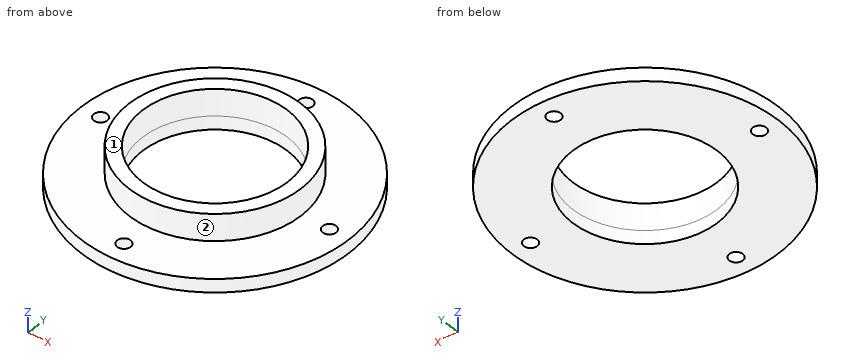
Autodesk Inventor part; units mm, degrees
ref_plane "YZ Plane" through (0, 0, 0) normal (1, 0, 0) x (0, 1, 0)
ref_plane "XZ Plane" through (0, 0, 0) normal (0, 1, 0) x (-1, 0, 0)
ref_plane "XY Plane" through (0, 0, 0) normal (0, 0, 1) x (1, 0, 0)
sketch "Boceto1" plane through (0, 0, 0) normal (0, 0, 1) x (1, 0, 0)
  circle A0 centre (0, 0) radius 16.26
  circle A1 centre (0, 0) radius 19.26
  dimension "d0" = 32.52
  dimension "d1" = 3
extrude "Extrusión1" add sketch "Boceto1" along normal blind 6
sketch "Boceto2" plane through (0, 0, 0) normal (0, 0, -1) x (-1, 0, 0)
  circle A0 centre (0, 0) radius 30
  circle A1 centre (0, 0) radius 16.26
  dimension "d4" = 60
extrude "Extrusión2" add sketch "Boceto2" along normal blind 3
sketch "Boceto3" plane through (0, 0, 0) normal (0, 0, 1) x (1, 0, 0)
  circle A0 centre (0, 0) radius 30
  circle A1 centre (0, 25.5) radius 1.5
  dimension "d7" = 3
  dimension "d8" = 25.5
  dimension "d9" = 60
extrude "Extrusión3" cut sketch "Boceto3" against normal blind 3 contours A1
pattern_circular "Patrón circular1" count 4 over 360 about axis through (0, 0, -10) along (0, 0, 1) of "Extrusión3"
properties part number "Acople N°1"
Can you work these out from the model? Positions are in its coordinate system, mm. Face numbers are marked on the shaded views. A direction names the side the tool comes from. Coordinates: 2 decimals unless noted, no trailing zeros. Write each loop counter-clockwise with the first axis right and the second up, starting at its lowest first coordinate (ties: lowest second). Pieces come first, ordered by that corner, then holes. Notation, with made-up numbers: (-24, -14.75) - (-15, -14.75) arc R19 ccw to (-15, 20.25) - close; hole circle Ø9 at (73, 30.5). An arc over 180 degrees is marked (long way). Return JSON: item names as keys, results as strings.
Q1. If we section it at C-C (x = 25.5): Please give me the cut outline in (y, z), then the cut area to 3 significant figures.
Computed values:
{"outline": "(-15.8, -3) - (-1.5, -3) - (-1.5, 0) - (-15.8, 0) - close; (1.5, -3) - (15.8, -3) - (15.8, 0) - (1.5, 0) - close", "area": "85.8 mm2"}
Q2. I'm going to push flat-ended pins straight in: pin 1 Ø3 at (x, z) = (13.5, -0.5) entering from +Y; pin 2 Ø6 at (x, y) = (18.5, 22) entering from +Z; pin 3 Ø12 at (x, y) = (11.5, -6.5) entering from +Z; pin 4 Ø5 at (y, z) = (5.5, -2) entering from +X. Where does each tip first touch, or does it pass through?
Computed values:
{"pin 1": "stops at y = 27.5", "pin 2": "stops at z = 0", "pin 3": "stops at z = 6", "pin 4": "stops at x = 29.85"}
Q3. On a 3-axis mill with a long thin cutter (end or side, diameter ignored), from which of +Z, -Z, +X, -X, +Y, -Y can I reach the whole of each face in a straight line? I mean the marked faces 1 and 2. Say none if no direction works.
Computed values:
{"face 1": "+Z, +X, -X, +Y, -Y", "face 2": "+Z"}
Q4. If we section it at A-A (x = 0): Please give me the cut outline in (y, z), then the cut area to 3 significant figures.
Computed values:
{"outline": "(-30, -3) - (-27, -3) - (-27, 0) - (-30, 0) - close; (-24, -3) - (-16.26, -3) - (-16.26, 6) - (-19.26, 6) - (-19.26, 0) - (-24, 0) - close; (16.26, -3) - (24, -3) - (24, 0) - (19.26, 0) - (19.26, 6) - (16.26, 6) - close; (27, -3) - (30, -3) - (30, 0) - (27, 0) - close", "area": "100 mm2"}
Q5. Please list where these lines run through material, in increasing order: L1, parallel to Y at x = 0, z = -1.9; L2, parallel to Y at x = -1, z = -0.25. Write a range as from..to.
Computed values:
{"L1": "y = -30..-27, -24..-16.26, 16.26..24, 27..30", "L2": "y = -29.98..-26.62, -24.38..-16.23, 16.23..24.38, 26.62..29.98"}
